from build123d import *

# Parameters (mm, degrees)
F0_W     = 6.8263569847
F0_H     = 1.6141139204
F1_DEPTH = 2
F2_DEPTH = 22
F4_DEPTH = 1.4
F5_W     = 1.2100687839
F5_H     = 1.0110005358
F6_DEPTH = 2


with BuildPart() as f1:
    # F0 (on Top) → F1 (new body)
    with BuildSketch(Plane.XY):
        with BuildLine():
            ThreePointArc((1.4161020408, -4.7952742372), (4.0050287267, -2.9932832973), (5, 0))
            ThreePointArc((5, 0), (3.9401994822, 3.0781208619), (1.2100687839, 4.8513640905))
            Line((1.2100687839, 4.8513640905), (1.2100687839, 4.0219067043))
            ThreePointArc((1.2100687839, 4.0219067043), (-4.1985994161, -0.1084571011), (1.4161020408, -3.9540681595))
            Line((1.4161020408, -3.9540681595), (1.4161020408, -4.7952742372))
        make_face()
        with Locations((0.043381704, -0.0145365484)):
            Rectangle(F0_W, F0_H, mode=Mode.SUBTRACT)
    extrude(amount=F1_DEPTH)

    # F0 (on Top) → F2 (join)
    with BuildSketch(Plane.XY):
        with BuildLine():
            Line((1.2100687839, 4.0219067043), (1.2100687839, 4.8513640905))
            ThreePointArc((1.2100687839, 4.8513640905), (-4.9988599757, -0.1067658356), (1.4161020408, -4.7952742372))
            Line((1.4161020408, -4.7952742372), (1.4161020408, -3.9540681595))
            ThreePointArc((1.4161020408, -3.9540681595), (-4.1985994161, -0.1084571011), (1.2100687839, 4.0219067043))
        make_face()
    extrude(amount=F2_DEPTH)

    # F3 (on face) → F4 (join)
    with BuildSketch(Plane.XY.offset(22)):
        with BuildLine():
            ThreePointArc((3.4046116017, -0.8115539672), (-3.4999864728, 0.0097308767), (3.409071597, 0.792610148))
            Line((3.409071597, 0.792610148), (4.9367772031, 0.792610148))
            ThreePointArc((4.9367772031, 0.792610148), (-4.9999907913, 0.0095961861), (4.933698426, -0.8115539672))
            Line((4.933698426, -0.8115539672), (3.4046116017, -0.8115539672))
        make_face()
    extrude(amount=F4_DEPTH)

    # F5 (on face) → F6 (cut)
    with BuildSketch(Plane.XY.offset(2)):
        with Locations((0.6050343919, 4.5274069722)):
            Rectangle(F5_W, F5_H)
    extrude(amount=F6_DEPTH, mode=Mode.SUBTRACT)


solid = f1.part
Model file for the job. Use its own axes, mm. A direction names the side the tool comes from. Give positions to 0.01 mm unless a question says otherwise; leave off trailing zeros. Loops run counter-clockwise (first coordinate to the right, second up) from the corner with the lowest first, then second, coordinate; pieces in that order, holes last.
1) Saw through at D-D (x = -2). Write the cut outline in (y, z).
2) Saw through at B-B (y = -2.5). Write the cut outline in (x, z).
3) Saw through at A-A (x = 1.75). Write the cut outline in (y, z).
4) Tool access for faces 1 (the flat face through (4, 0.793, 23)), 2 (the cylindrical face through (-4.194, -0.219, 11.86)), 3 (the flat face through (1.21, 4.4, 12.9)), 4 (the flat face through (0, -0.822, 1)): list every direction of +Z, -Z, +X, -X, +Y, -Y with a clear straight run to the whole face (end or side of a thin tool).
5) Pull direction X, two halves, no side cores. Call faces 5 (the flat face through (1.416, -4.4, 11.9)), 6 (the cylindrical face through (-3.5, -0.1, 22.7)), 7 (the flat face through (3.457, 0, 1)), 8 (the flat face through (0.6, 4.5, 4)): +X half, -X half, draft (parallel to the pull), parting line (faces both ways), or undercut.
6) Flat gauge pins, fed straight in: pin 1 Ø1 at (x, z) = (-1, 1) entering from +Y; pin 2 Ø2 at (x, y) = (0, 1) entering from +Z; pin 3 Ø1.1 at (x, z) = (4, 23) entering from +Y. Where does each tip first touch, or does it go through?
7) Wall check: line 1 (Y direction, x = 0, z = 22.8); line 2 (Y direction, x = 0, z = 10.5); line 3 (Z direction, x = 0.25, y = 3.75). Give the ranges that are in metal, low to high.
8) Saw through at C-C (x = 3.75). Write the cut outline in (y, z).
Answer block:
1. outline: (-4.58, 0) - (-0.82, 0) - (-0.82, 2) - (-3.69, 2) - (-3.69, 22) - (-2.87, 22) - (-2.87, 23.4) - (-4.58, 23.4) - close; (0.79, 0) - (4.58, 0) - (4.58, 23.4) - (2.87, 23.4) - (2.87, 22) - (3.69, 22) - (3.69, 2) - (0.79, 2) - close
2. outline: (-4.33, 0) - (4.33, 0) - (4.33, 2) - (-3.37, 2) - (-3.37, 22) - (-2.45, 22) - (-2.45, 23.4) - (-4.33, 23.4) - close; (2.45, 22) - (4.33, 22) - (4.33, 23.4) - (2.45, 23.4) - close
3. outline: (-4.68, 0) - (-0.82, 0) - (-0.82, 2) - (-4.68, 2) - close; (-4.68, 22) - (-3.03, 22) - (-3.03, 23.4) - (-4.68, 23.4) - close; (0.79, 0) - (4.68, 0) - (4.68, 2) - (0.79, 2) - close; (3.03, 22) - (4.68, 22) - (4.68, 23.4) - (3.03, 23.4) - close
4. face 1: +Z, +X
4. face 2: none
4. face 3: +X, +Y
4. face 4: +Z, -Z
5. face 5: +X half
5. face 6: undercut
5. face 7: undercut
5. face 8: draft
6. pin 1: stops at y = 4.97
6. pin 2: stops at z = 2
6. pin 3: stops at y = 3.62
7. line 1: y = -5 to -3.5, 3.5 to 5
7. line 2: y = -5 to -4.2, 4.2 to 5
7. line 3: z = 0 to 2, 22 to 23.4
8. outline: (-3.31, 0) - (3.31, 0) - (3.31, 2) - (-3.31, 2) - close; (-3.31, 22) - (-0.81, 22) - (-0.81, 23.4) - (-3.31, 23.4) - close; (0.79, 22) - (3.31, 22) - (3.31, 23.4) - (0.79, 23.4) - close
